```python
from build123d import *

# Parameters (mm, degrees)
SKETCH1_R           = 1
SKETCH1_R_2         = 2
BOSS_EXTRUDE1_DEPTH = 3


with BuildPart() as part:
    # Sketch1 → Boss-Extrude1 (new body)
    with BuildSketch(Plane(origin=(0, 0, 0), x_dir=(0, 0, -1), z_dir=(1, 0, 0))):
        with BuildLine():
            ThreePointArc((376.492857784, -15.618533096), (384.381466904, -12.492857784), (387.507142216, -20.381466904))
            Line((387.507142216, -20.381466904), (369.942371147, -61))
            Line((369.942371147, -61), (366, -61))
            Line((366, -61), (54.561190838, -61))
            Line((54.561190838, -61), (-4.166215043, -4.317713772))
            ThreePointArc((-4.166215043, -4.317713772), (-4.317713772, 4.166215043), (4.166215043, 4.317713772))
            Line((4.166215043, 4.317713772), (59.42275477, -49))
            Line((59.42275477, -49), (362.057628853, -49))
            Line((362.057628853, -49), (376.492857784, -15.618533096))
        make_face()
        with Locations((382, -18)):
            Circle(SKETCH1_R, mode=Mode.SUBTRACT)
        with Locations((366, -55)):
            Circle(SKETCH1_R_2, mode=Mode.SUBTRACT)
        with Locations((303, -55)):
            Circle(SKETCH1_R_2, mode=Mode.SUBTRACT)
        with Locations((241, -55)):
            Circle(SKETCH1_R_2, mode=Mode.SUBTRACT)
        with Locations((178, -55)):
            Circle(SKETCH1_R_2, mode=Mode.SUBTRACT)
        with Locations((116, -55)):
            Circle(SKETCH1_R_2, mode=Mode.SUBTRACT)
        with Locations((57, -55)):
            Circle(SKETCH1_R_2, mode=Mode.SUBTRACT)
        Circle(SKETCH1_R_2, mode=Mode.SUBTRACT)
    extrude(amount=BOSS_EXTRUDE1_DEPTH)


solid = part.part
```
The listing builds one solid part. Answer for the finished solid, in the listing's coordinates (mm). Round coordinates to 2 decimals unless told otherwise and drop trailing zeros. Loops run counter-clockwise (first coordinate to the right, second up) from the corner with the lowest first, then second, coordinate; pieces in that order, holes last.
Q1. Section C-C, the plane z = -294.5 is taken. Determine the outline of the cut face in (x, y), then the cut area to 3 significant figures.
Q2. Find the intervals of material crossed by line 1 (Y direction, x = 0.45, z = -205.5); line 2 (Z direction, x = 1.5, y = -31.5); line 3 (Z direction, x = 0.65, y = -14.5), in increasing order.
Q3. Given pin 1 Ø3 at (y, z) = (-18, -382) entering from -X; pin 2 Ø1 at (x, y) = (2, -47.5) entering from -Z; pin 3 Ø3.5 at (y, z) = (-55, -366) entering from +X; pin 4 Ø0.9 at (x, z) = (2, -212.5) entering from +Y, each flat-ended and moving along its own axis, determine where each tip first touches the part or whether it passes through.
Q4. Section B-B, the plane x = 0.9 is taken. Count the separate pieces of the cut face and the enclosed holes in it, then the cut area to 3 significant figures.
Q5. Section D-D, the plane z = -41.5 is taken. Determine the outline of the cut face in (x, y).
Q6. For a pull along Z with two mould halves and no side action, classify faces 1 (the face through (1.479, -32.543, -369.174)), 2 (the face through (3, -50, -192)), 3 (the face through (1.48, -21.97, -31.41)), 4 (the face through (1.479, -33.056, -25.609)) as released by +Z, released by -Z, zero draft, split by the parting line, or undercut.
Q7. Section A-A, the plane y = -43.5 is taken. Determine the outline of the cut face in (x, z), then the cut area to 3 significant figures.
Completed:
1. outline: (0, -61) - (3, -61) - (3, -49) - (0, -49) - close
1. area: 36.0 mm2
2. line 1: y = -61 to -49
2. line 2: z = -382.7 to -369.63, -41.29 to -24
2. line 3: z = -386.87 to -377.13, -23.67 to -6.38
3. pin 1: stops at x = 0
3. pin 2: stops at z = -376
3. pin 3: passes through
3. pin 4: stops at y = -49
4. separate pieces: 1
4. enclosed holes: 8
4. area: 5,160 mm2
5. outline: (0, -48.39) - (3, -48.39) - (3, -31.71) - (0, -31.71) - close
6. face 1: undercut
6. face 2: zero draft
6. face 3: undercut
6. face 4: released by +Z
7. outline: (0, -377.51) - (3, -377.51) - (3, -364.44) - (0, -364.44) - close; (0, -53.72) - (3, -53.72) - (3, -36.43) - (0, -36.43) - close
7. area: 91.1 mm2
